Here's how the part is built. I have some questions about the finished solid (model axes, mm). Face numbers are marked on the shaded views. A direction names the side the tool comes from. Coordinates: 2 decimals unless noted, no trailing zeros. Write each loop counter-clockwise with the first axis right and the second up, starting at its lowest first coordinate (ties: lowest second). Pieces come first, ordered by that corner, then holes. Notation, with made-up numbers: M 7.25,79.25 L 31.25,79.25 A14 ccw 31.25,86.25 Z; hole C 30.25,41.5 d4. An arc over 180 degrees is marked long. Use one line per item in the form item = value. Start each with the question number.
1. On a 3-axis mill with a long thin cutter (end or side, diameter ignored), from which of +Z, -Z, +X, -X, +Y, -Y can I reach the whole of each face in a straight line? I mean the marked faces 1, 2, 3 and 4. Say none if no direction works.
2. I want a section at A-A, the plane x = 0. List the corners of the cut face in (y, z) for me, plus the area to 4 significant figures.
3. I want a section at D-D, the plane y = 13. List the corners of the cut face in (x, z) for me, plus the area to 3 significant figures.
4. I want a section at C-C, the plane z = 8.5. Count the separate pieces of the cut face and the enclosed holes in it, plus the area to 3 significant figures.
5. Please list where these lines run through material, in increasing order: line 1 along Z through (x, y) = (6, 7); line 2 along X through (y, z) = (-3, 1.25); line 3 along Y through (x, z) = (9, 2.75). Write a range as [from, to].
6. I'm going to push flat-ended pins straight in: pin 1 Ø0.9 at (x, z) = (15, 4.5) entering from +Y; pin 2 Ø8 at (x, y) = (-6.5, -0.5) entering from +Z; pin 3 Ø1.6 at (x, z) = (-15, 5) entering from -Y; pin 4 Ø3.5 at (y, z) = (15.5, 4.5) entering from -X. Where does each tip first touch, or does it pass through?
from build123d import *

# Parameters (mm, degrees)
SKETCH_1_R          = 14
EXTRUDE_2_DEPTH     = 10
SKETCH_2_R          = 10.75
CUT_EXTRUDE_1_DEPTH = 4
SKETCH_3_R          = 1.5
CUT_EXTRUDE_2_DEPTH = 10
SKETCH_4_R          = 3.75
CUT_EXTRUDE_3_DEPTH = 1


with BuildPart() as part:
    # 草圖1 → 填料-伸長2 (new body)
    with BuildSketch(Plane.XY):
        Circle(SKETCH_1_R)
        with BuildLine():
            Line((-4.011695199, 16.519875957), (-4.011695199, 13.412915478))
            ThreePointArc((-4.011695199, 13.412915478), (-1.827366691, 13.880228059), (0.403482024, 13.994184587))
            Line((0.403482024, 13.994184587), (-0.40065852, 16.995277954))
            ThreePointArc((-0.40065852, 16.995277954), (-2.218945268, 16.854562643), (-4.011695199, 16.519875957))
        make_face()
        with BuildLine():
            Line((4.785708024, 16.312479846), (3.232227785, 13.621773143))
            ThreePointArc((3.232227785, 13.621773143), (5.357568053, 12.934313455), (7.346517976, 11.917578346))
            Line((7.346517976, 11.917578346), (8.15065852, 14.918671713))
            ThreePointArc((8.15065852, 14.918671713), (6.50561835, 15.705952053), (4.785708024, 16.312479846))
        make_face()
        with BuildLine():
            Line((12.300784646, 11.734167933), (9.610077944, 10.180687694))
            ThreePointArc((9.610077944, 10.180687694), (11.106946764, 8.522660006), (12.32106037, 6.647666611))
            Line((12.32106037, 6.647666611), (14.518013193, 8.844619434))
            ThreePointArc((14.518013193, 8.844619434), (13.487006785, 10.348944293), (12.300784646, 11.734167933))
        make_face()
        with BuildLine():
            Line((16.519875957, 4.011695199), (13.412915478, 4.011695199))
            ThreePointArc((13.412915478, 4.011695199), (13.852451348, 2.027212779), (14, 0))
            ThreePointArc((14, 0), (13.998546071, -0.201761965), (13.994184587, -0.403482024))
            Line((13.994184587, -0.403482024), (16.995277954, 0.40065852))
            ThreePointArc((16.995277954, 0.40065852), (16.854562643, 2.218945268), (16.519875957, 4.011695199))
        make_face()
        with BuildLine():
            Line((16.312479846, -4.785708024), (13.621773143, -3.232227785))
            ThreePointArc((13.621773143, -3.232227785), (12.934313455, -5.357568053), (11.917578346, -7.346517976))
            Line((11.917578346, -7.346517976), (14.918671713, -8.15065852))
            ThreePointArc((14.918671713, -8.15065852), (15.705952053, -6.50561835), (16.312479846, -4.785708024))
        make_face()
        with BuildLine():
            ThreePointArc((10.180687694, -9.610077944), (8.522660006, -11.106946764), (6.647666611, -12.32106037))
            Line((6.647666611, -12.32106037), (8.844619434, -14.518013193))
            ThreePointArc((8.844619434, -14.518013193), (10.348944293, -13.487006785), (11.734167933, -12.300784646))
            Line((11.734167933, -12.300784646), (10.180687694, -9.610077944))
        make_face()
        with BuildLine():
            ThreePointArc((4.011695199, -13.412915478), (1.827366691, -13.880228059), (-0.403482024, -13.994184587))
            Line((-0.403482024, -13.994184587), (0.40065852, -16.995277954))
            ThreePointArc((0.40065852, -16.995277954), (2.218945268, -16.854562643), (4.011695199, -16.519875957))
            Line((4.011695199, -16.519875957), (4.011695199, -13.412915478))
        make_face()
        with BuildLine():
            ThreePointArc((-3.232227785, -13.621773143), (-5.357568053, -12.934313455), (-7.346517976, -11.917578346))
            Line((-7.346517976, -11.917578346), (-8.15065852, -14.918671713))
            ThreePointArc((-8.15065852, -14.918671713), (-6.50561835, -15.705952053), (-4.785708024, -16.312479846))
            Line((-4.785708024, -16.312479846), (-3.232227785, -13.621773143))
        make_face()
        with BuildLine():
            ThreePointArc((-9.610077944, -10.180687694), (-11.106946764, -8.522660006), (-12.32106037, -6.647666611))
            Line((-12.32106037, -6.647666611), (-14.518013193, -8.844619434))
            ThreePointArc((-14.518013193, -8.844619434), (-13.487006785, -10.348944293), (-12.300784646, -11.734167933))
            Line((-12.300784646, -11.734167933), (-9.610077944, -10.180687694))
        make_face()
        with BuildLine():
            ThreePointArc((-13.412915478, -4.011695199), (-13.880228059, -1.827366691), (-13.994184587, 0.403482024))
            Line((-13.994184587, 0.403482024), (-16.995277954, -0.40065852))
            ThreePointArc((-16.995277954, -0.40065852), (-16.854562643, -2.218945268), (-16.519875957, -4.011695199))
            Line((-16.519875957, -4.011695199), (-13.412915478, -4.011695199))
        make_face()
        with BuildLine():
            ThreePointArc((-13.621773143, 3.232227785), (-12.934313455, 5.357568053), (-11.917578346, 7.346517976))
            Line((-11.917578346, 7.346517976), (-14.918671713, 8.15065852))
            ThreePointArc((-14.918671713, 8.15065852), (-15.705952053, 6.50561835), (-16.312479846, 4.785708024))
            Line((-16.312479846, 4.785708024), (-13.621773143, 3.232227785))
        make_face()
        with BuildLine():
            Line((-11.734167933, 12.300784646), (-10.180687694, 9.610077944))
            ThreePointArc((-10.180687694, 9.610077944), (-8.522660006, 11.106946764), (-6.647666611, 12.32106037))
            Line((-6.647666611, 12.32106037), (-8.844619434, 14.518013193))
            ThreePointArc((-8.844619434, 14.518013193), (-10.348944293, 13.487006785), (-11.734167933, 12.300784646))
        make_face()
    extrude(amount=EXTRUDE_2_DEPTH)

    # 草圖2 → 除料-伸長1 (cut)
    with BuildSketch(Plane(origin=(0, 0, 0), x_dir=(-1, 0, 0), z_dir=(0, 0, -1))):
        Circle(SKETCH_2_R)
    extrude(amount=-CUT_EXTRUDE_1_DEPTH, mode=Mode.SUBTRACT)

    # 草圖3 → 除料-伸長2 (cut)
    with BuildSketch(Plane.XY.offset(10)):
        with Locations((-7.5, 0)):
            Circle(SKETCH_3_R)
        with Locations((7.5, 0)):
            Circle(SKETCH_3_R)
        with Locations((0, 7.5)):
            Circle(SKETCH_3_R)
        with Locations((0, -7.5)):
            Circle(SKETCH_3_R)
    extrude(amount=-CUT_EXTRUDE_2_DEPTH, mode=Mode.SUBTRACT)

    # 草圖4 → 除料-伸長3 (cut)
    with BuildSketch(Plane(origin=(0, 0, 4), x_dir=(-1, 0, 0), z_dir=(0, 0, -1))):
        Circle(SKETCH_4_R)
    extrude(amount=-CUT_EXTRUDE_3_DEPTH, mode=Mode.SUBTRACT)


solid = part.part
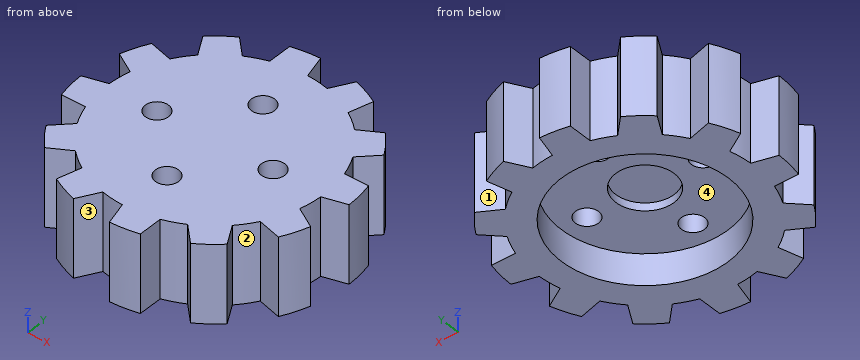
Answer list:
q1.face_1 = +Z, -Z, +Y
q1.face_2 = +Z, -Z
q1.face_3 = +Z, -Z, -Y
q1.face_4 = -Z
q2.outline = M -15.5,0 L -10.75,0 L -10.75,4 L -9,4 L -9,10 L -15.5,10 Z; M -6,4 L -3.75,4 L -3.75,5 L 3.75,5 L 3.75,4 L 6,4 L 6,10 L -6,10 Z; M 9,4 L 10.75,4 L 10.75,0 L 15.5,0 L 15.5,10 L 9,10 Z
q2.area = 180.5 mm²
q3.outline = M -10.95,0 L -7.33,0 L -7.33,10 L -10.95,10 Z; M -5.2,0 L 7.64,0 L 7.64,10 L -5.2,10 Z
q3.area = 165 mm²
q4.separate_pieces = 1
q4.enclosed_holes = 4
q4.area = 734 mm²
q5.line_1 = [4, 10]
q5.line_2 = [-16.73, -10.32], [10.32, 13.67]
q5.line_3 = [-14.42, -5.88], [5.88, 10.72]
q6.pin_1 = 4.01
q6.pin_2 = 10
q6.pin_3 = -9.35
q6.pin_4 = -10
